```python
from build123d import *

# Parameters (mm, degrees)
SKETCH1_R   = 1.5
BOARD_DEPTH = 1.6
FILLET1_R   = 2.56


with BuildPart() as part:
    # Sketch1 → Board (new body)
    with BuildSketch(Plane.XY):
        Polygon((20, 20), (117, 20), (117, 137), (106, 137), (106, 75.46), (31, 75.46), (31, 137), (20, 137), align=None)
        with Locations((22.6657, 134.46)):
            Circle(SKETCH1_R, mode=Mode.SUBTRACT)
        with Locations((114.3343, 134.46)):
            Circle(SKETCH1_R, mode=Mode.SUBTRACT)
        with Locations((22.6657, 73.5)):
            Circle(SKETCH1_R, mode=Mode.SUBTRACT)
        with Locations((114.3343, 73.5)):
            Circle(SKETCH1_R, mode=Mode.SUBTRACT)
    extrude(amount=BOARD_DEPTH)

    # Fillet1
    fillet1_edges = [part.edges().sort_by_distance(p)[0] for p in [
        (20, 137, 0.8),
        (31, 137, 0.8),
        (31, 75.46, 0.8),
        (106, 75.46, 0.8),
        (106, 137, 0.8),
        (117, 137, 0.8),
        (117, 20, 0.8),
        (20, 20, 0.8),
    ]]
    fillet(fillet1_edges, radius=FILLET1_R)


solid = part.part
```
Geometry: final body of the model. Coordinates: model frame, mm. A direction names the side the tool comes from. Give positions to 0.01 mm unless a question says otherwise; leave off trailing zeros. Loops run counter-clockwise (first coordinate to the right, second up) from the corner with the lowest first, then second, coordinate; pieces in that order, holes last. Notation, with made-up numbers: (70.5, 29) - (99.5, 29) arc R11 cw to (99.5, 47) - close; hole circle Ø10 at (71.25, 61.5). An arc over 180 degrees is marked (long way). Answer as CSV lines item,"result". Start each with the question number.
(1) Ray query, line 1 along X through (y, z) = (73.5, 0.8); line 2 along X through (y, z) = (134.46, 0.5); line 3 along X through (y, z) = (87.5, 0.4). Return the intervals inside material, ascending. Write a range as [from, to].
(2) Section query A-A (y = 127). Output: boundary loops of the cut face in (x, z), and give its area (3 significant figures).
(3) Section query C-C (y = 73.5). Output: boundary loops of the cut face in (x, z), and give its area (3 significant figures).
(4) Reachability of faces 5 (the face through (20.8, 20.7, 0.8)), 6 (the face through (106.8, 136.3, 0.8)) from +Z, -Z, +X, -X, +Y, -Y: full face, straight path, thin tool, end or side. Return the list, or none.
(5) Section query D-D (x = 74). Output: boundary loops of the cut face in (y, z), and give its area (3 significant figures).
(6) Section query B-B (z = 1.35). Output: boundary loops of the cut face in (x, y), and give its area (3 significant figures).
(7) Mould query, pull axis X, two halves, no side actions, for faces 1 (the face through (116.2, 20.7, 0.8)), 2 (the face through (115.765, 73.951, 0.789)), 3 (the face through (20.7, 136.2, 0.8)), 4 (the face through (68, 53, 1.6)). Classes: +X half, -X half, draft (parallel to the pull), parting line (faces both ways), or undercut.
Worked answers:
1,line 1,"x = [20, 21.17], [24.17, 112.83], [115.83, 117]"
1,line 2,"x = [20, 21.17], [24.17, 31], [106, 112.83], [115.83, 117]"
1,line 3,"x = [20, 31], [106, 117]"
2,outline,"(20, 0) - (31, 0) - (31, 1.6) - (20, 1.6) - close; (106, 0) - (117, 0) - (117, 1.6) - (106, 1.6) - close"
2,area,"35.2 mm^2"
3,outline,"(20, 0) - (21.17, 0) - (21.17, 1.6) - (20, 1.6) - close; (24.17, 0) - (112.83, 0) - (112.83, 1.6) - (24.17, 1.6) - close; (115.83, 0) - (117, 0) - (117, 1.6) - (115.83, 1.6) - close"
3,area,"146 mm^2"
4,face 5,"+Z, -Z, -X, -Y"
4,face 6,"+Z, -Z, +Y"
5,outline,"(20, 0) - (75.46, 0) - (75.46, 1.6) - (20, 1.6) - close"
5,area,"88.7 mm^2"
6,outline,"(20, 22.56) arc R2.56 ccw to (22.56, 20) - (114.44, 20) arc R2.56 ccw to (117, 22.56) - (117, 134.44) arc R2.56 ccw to (114.44, 137) - (108.56, 137) arc R2.56 ccw to (106, 134.44) - (106, 78.02) arc R2.56 cw to (103.44, 75.46) - (33.56, 75.46) arc R2.56 cw to (31, 78.02) - (31, 134.44) arc R2.56 ccw to (28.44, 137) - (22.56, 137) arc R2.56 ccw to (20, 134.44) - close; hole circle Ø3 at (22.67, 73.5); hole circle Ø3 at (22.67, 134.46); hole circle Ø3 at (114.33, 73.5); hole circle Ø3 at (114.33, 134.46)"
6,area,"6,700 mm^2"
7,face 1,"+X half"
7,face 2,"undercut"
7,face 3,"-X half"
7,face 4,"draft"
